The model under review builds one solid part; all positions refer to its coordinate system, in mm. Coordinates: 2 decimals unless noted, no trailing zeros. Loops run counter-clockwise (first coordinate to the right, second up) from the corner with the lowest first, then second, coordinate; pieces in that order, holes last. Notation, with made-up numbers: M -22.5,-12 L 33.5,-12 A20 cw 33.5,23 Z; hole C -40,40.5 d9. An arc over 180 degrees is marked long. Use CSV: the item, a comma, the result in double quotes. Start each with the question number.
1. Add section C-C, the plane x = 42. Write out the cut boundary in (y, z), then the cut area to 3 significant figures.
2. Draft analysis for pull direction X (two halves, no side actions). For faces 1 (the cylindrical face through (-52.5, 0.99, 5.41)), 2 (the cylindrical face through (54.352, 0.986, 0.548)), 3 (the cylindrical face through (0.742, 0.986, -6.124)), state which applies: +X half, -X half, draft (parallel to the pull), parting line (faces both ways), or undercut.
3. For L1, parallel to X at y = 1.8, z = 25; L2, parallel to Z at x = -51, y = 0.6; L3, parallel to Z at x = -40, y = 1.55, list the stretches that pass through material, from the lowest coordinate up.
4. Add section A-A, the plane x = -51. Write out the cut boundary in (y, z), then the cut area to 3 significant figures.
5. Add section B-B, the plane x = -22. Write out the cut boundary in (y, z).
from build123d import *

# Parameters (mm, degrees)
SKETCH_1_R      = 1.5
EXTRUDE_1_DEPTH = 2


with BuildPart() as part:
    # Эскиз1 → Бобышка-Вытянуть1 (new body)
    with BuildSketch(Plane(origin=(0, 0, 0), x_dir=(1, 0, 0), z_dir=(0, 1, 0))):
        with BuildLine():
            Line((-55, -2.410684892), (-55, -27.589315108))
            ThreePointArc((-55, -27.589315108), (-54.333959816, -29.474157695), (-52.631578947, -30.52207968))
            ThreePointArc((-52.631578947, -30.52207968), (0, -36.125032035), (52.631578947, -30.52207968))
            ThreePointArc((52.631578947, -30.52207968), (54.333959816, -29.474157695), (55, -27.589315108))
            Line((55, -27.589315108), (55, -2.410684892))
            ThreePointArc((55, -2.410684892), (54.333959816, -0.525842305), (52.631578947, 0.52207968))
            ThreePointArc((52.631578947, 0.52207968), (0, 6.125032035), (-52.631578947, 0.52207968))
            ThreePointArc((-52.631578947, 0.52207968), (-54.333959816, -0.525842305), (-55, -2.410684892))
        make_face()
        with Locations((-51, -5.47792032)):
            Circle(SKETCH_1_R, mode=Mode.SUBTRACT)
        with Locations((-51, -24.52207968)):
            Circle(SKETCH_1_R, mode=Mode.SUBTRACT)
        with Locations((51, -5.47792032)):
            Circle(SKETCH_1_R, mode=Mode.SUBTRACT)
        with Locations((51, -24.52207968)):
            Circle(SKETCH_1_R, mode=Mode.SUBTRACT)
    extrude(amount=EXTRUDE_1_DEPTH)


solid = part.part
Computed:
1,outline,"M 0,-2.57 L 2,-2.57 L 2,32.57 L 0,32.57 Z"
1,area,"70.3 mm^2"
2,face 1,"undercut"
2,face 2,"+X half"
2,face 3,"parting line"
3,L1,"x = -55 to -52.42, -49.58 to 49.58, 52.42 to 55"
3,L2,"z = -0.87 to 3.98, 6.98 to 23.02, 26.02 to 30.87"
3,L3,"z = -2.9 to 32.9"
4,outline,"M 0,-0.87 L 2,-0.87 L 2,3.98 L 0,3.98 Z; M 0,6.98 L 2,6.98 L 2,23.02 L 0,23.02 Z; M 0,26.02 L 2,26.02 L 2,30.87 L 0,30.87 Z"
4,area,"51.5 mm^2"
5,outline,"M 0,-5.16 L 2,-5.16 L 2,35.16 L 0,35.16 Z"
